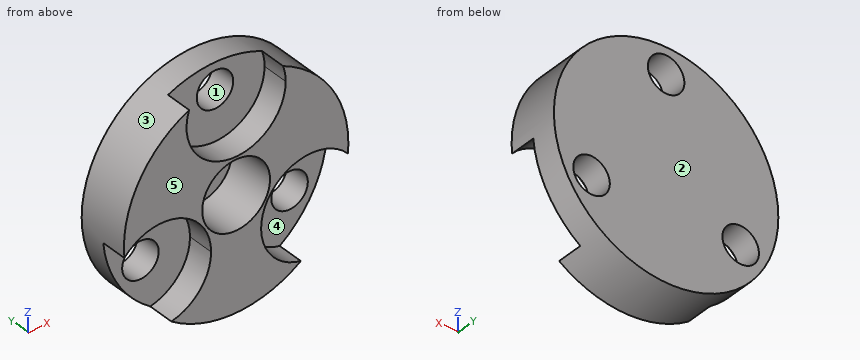
from build123d import *

# Parameters (mm, degrees)
F0_R     = 4.3
F1_DEPTH = 2
F2_R     = 0.7
F3_DEPTH = 1
F4_DEPTH = 2
F5_R     = 1.3
F6_DEPTH = 1.8


with BuildPart() as f1:
    # F0 (on Front) → F1 (new body)
    with BuildSketch(Plane.XZ):
        Circle(F0_R)
    extrude(amount=F1_DEPTH)

    # F2 (on face) → F3 (cut)
    with BuildSketch(Plane.XZ.offset(2)):
        with BuildLine():
            ThreePointArc((-1.8012564485, 3.9045454545), (-0.3062782622, 1.4248483725), (1.9, 3.3))
            ThreePointArc((1.9, 3.3), (1.8751516275, 3.6062782622), (1.8012564485, 3.9045454545))
            ThreePointArc((1.8012564485, 3.9045454545), (0, 4.3), (-1.8012564485, 3.9045454545))
        make_face()
        with Locations((0, 3.3)):
            Circle(F2_R, mode=Mode.SUBTRACT)
        with BuildLine():
            ThreePointArc((-0.9578838325, -1.65), (-2.1855527744, 0.1270680765), (-4.2820637781, -0.3923388841))
            ThreePointArc((-4.2820637781, -0.3923388841), (-3.7239092363, -2.15), (-2.4808073296, -3.5122065704))
            ThreePointArc((-2.4808073296, -3.5122065704), (-1.3870940182, -2.8528205694), (-0.9578838325, -1.65))
        make_face()
        with Locations((-2.8578838325, -1.65)):
            Circle(F2_R, mode=Mode.SUBTRACT)
        with BuildLine():
            ThreePointArc((2.4808073296, -3.5122065704), (3.7239092363, -2.15), (4.2820637781, -0.3923388841))
            ThreePointArc((4.2820637781, -0.3923388841), (1.2124355653, -0.7), (2.4808073296, -3.5122065704))
        make_face()
        with Locations((2.8578838325, -1.65)):
            Circle(F2_R, mode=Mode.SUBTRACT)
    extrude(amount=-F3_DEPTH, mode=Mode.SUBTRACT)

    # F4 (cut): faces of the model
    f4_faces = [f1.faces().sort_by_distance(p)[0] for p in [
        (0, -2, 3.3),
        (-2.8578838325, -2, -1.65),
        (2.8578838325, -2, -1.65),
    ]]
    extrude(f4_faces, amount=-F4_DEPTH, mode=Mode.SUBTRACT)

    # F5 (on face) → F6 (cut)
    with BuildSketch(Plane.XZ.offset(2)):
        Circle(F5_R)
    extrude(amount=-F6_DEPTH, mode=Mode.SUBTRACT)


solid = f1.part
Design review of the part built by this model. Coordinates are the model's own, in mm. Face numbers are marked on the shaded views. A direction names the side the tool comes from. Coordinates: 2 decimals unless noted, no trailing zeros. Loops run counter-clockwise (first coordinate to the right, second up) from the corner with the lowest first, then second, coordinate; pieces in that order, holes last. Notation, with made-up numbers: (44, 79) -> (60, 79) arc R25 cw to (60, 114) -> close; hole circle Ø10 at (70, 50.25). An arc over 180 degrees is marked (long way). Use a Markdown table: item, result. Add a question column.
Item 1: We need section C-C, the plane z = 3.75. Write out the cut boundary in (x, y), and give its area (3 significant figures).
Item 2: Wall thickness on L1, parallel to Z at x = 0, y = -0.55; L2, parallel to X at y = -0.5, z = -1.5; L3, parallel to Y at x = 0.25, z = -0.5: over which ranges is each line inside the solid? List them lowest first. Write a range as from..to.
Item 3: We need section B-B, the plane y = -0.8. Write out the cut boundary in (x, z).
Item 4: Machinability: for the marked faces 4 and 5, which of the approach directions +Z, -Z, +X, -X, +Y, -Y give a long, thin tool a straight path to every point of the face, cutting with its end or side? Answer none if there is none.
Item 5: We need section D-D, the plane y = -1.85. Write out the cut boundary in (x, z), and give its area (3 significant figures).
Item 6: Clearance check with flat-ended pins moving along their axes: P1, Ø2, axis at x = -2.86, z = -1.65, coming from the -Y side; P2, Ø1, axis at y = -1.5, z = 2, coming from the -X side. State where each tip first meets the part, or that it passes through.
Item 7: The part is to be moulded in two halves that separate along X. For the marked faces 1, 2 and 3, say which applies: +X half, -X half, draft (parallel to the pull), parting line (faces both ways), or undercut.
Item 8: We need section A-A, the plane x = 0. Write out the cut boundary in (y, z), and give its area (3 significant figures).
Numbers:
| question | item | result |
|---|---|---|
| 1 | outline | (-2.1, -2) -> (-1.85, -2) -> (-1.85, -1) -> (-0.54, -1) -> (-0.54, 0) -> (-2.1, 0) -> close; (0.54, -1) -> (1.85, -1) -> (1.85, -2) -> (2.1, -2) -> (2.1, 0) -> (0.54, 0) -> close |
| 1 | area | 3.65 mm^2 |
| 2 | L1 | z = -4.3..-1.3, 1.3..2.6, 4..4.3 |
| 2 | L2 | x = -4.03..-3.54, -2.17..2.17, 3.54..4.03 |
| 2 | L3 | y = -0.2..0 |
| 3 | outline | circle Ø8.6 at (0, 0); hole circle Ø1.4 at (-2.86, -1.65); hole circle Ø2.6 at (0, 0); hole circle Ø1.4 at (0, 3.3); hole circle Ø1.4 at (2.86, -1.65) |
| 4 | face 4 | -Y |
| 4 | face 5 | +Z, -Z, +X, -X, -Y |
| 5 | outline | (-4.28, -0.39) arc R1.9 cw (long way) to (-2.48, -3.51) arc R4.3 ccw to (2.48, -3.51) arc R1.9 cw (long way) to (4.28, -0.39) arc R4.3 ccw to (1.8, 3.9) arc R1.9 cw (long way) to (-1.8, 3.9) arc R4.3 ccw to start; hole circle Ø2.6 at (0, 0) |
| 5 | area | 26.1 mm^2 |
| 6 | P1 | stops at y = -1 |
| 6 | P2 | stops at x = -4.03 |
| 7 | face 1 | undercut |
| 7 | face 2 | draft |
| 7 | face 3 | parting line |
| 8 | outline | (-2, -4.3) -> (0, -4.3) -> (0, 2.6) -> (-1, 2.6) -> (-1, 1.4) -> (-2, 1.4) -> (-2, 1.3) -> (-0.2, 1.3) -> (-0.2, -1.3) -> (-2, -1.3) -> close; (-1, 4) -> (0, 4) -> (0, 4.3) -> (-1, 4.3) -> close |
| 8 | area | 8.22 mm^2 |
